Source: CAD feature listing. Evaluate the final solid. Frame: model axes, mm. A direction names the side the tool comes from. Coordinates: 2 decimals unless noted, no trailing zeros. Loops run counter-clockwise (first coordinate to the right, second up) from the corner with the lowest first, then second, coordinate; pieces in that order, holes last.
Item 1: Pin query (flat end, axial travel): pin 1 Ø3 at (y, z) = (-5.5, -1.5) entering from -X; pin 2 Ø12 at (x, y) = (18.5, -10) entering from +Z; pin 3 Ø0.8 at (x, z) = (3.5, 3.5) entering from -Y; pin 4 Ø1.5 at (x, z) = (5.5, -1) entering from +Y. Return the tip coordinate at first contact, or that it passes through.
Item 2: Section query A-A, the plane y = 12.25. Return the cut outline in (x, z).
Item 3: Pull-direction query (X, two-part tool) for faces 1 (the flat face through (30, -3, 6.8)), 2 (the flat face through (0, 0, 0)), 3 (the flat face through (11.091, -8.787, -5.666)); classes: +X half, -X half, draft (parallel to the pull), parting line (faces both ways), or undercut.
Item 4: Section query B-B, the plane z = 4. Return the cut outline in (x, y).
Item 5: Reachability of faces 4 (the flat face through (15, -3, -6.8)), 5 (the flat face through (14, -5, -4.5)), 6 (the flat face through (2, -1, -5.3)), 7 (the flat face through (13, -1, 5.3)), 8 (the flat face through (4, 5.3, 2)) from +Z, -Z, +X, -X, +Y, -Y: full face, straight path, thin tool, end or side. Return the list, or none.
Item 6: Line query: probe 1 along X at (y, z) = (9, -3.25); probe 2 along X at (y, z) = (6.25, 1); probe 3 along X at (y, z) = (-1, 3.25). Output: solid intervals per line, ascending.
Item 7: Section query C-C, the plane y = -11.5. Return the cut outline in (x, z), then the cut area to 3 significant figures.
```python
from build123d import *

# Parameters (mm, degrees)
PAD_DEPTH            = 31
SKETCH001_W          = 11
SKETCH001_H          = 28.2
POCKET_DEPTH         = 10.6
SKETCH002_R          = 3
PAD001_DEPTH         = 3.8
SKETCH003_R          = 1.7
PAD002_DEPTH         = 4.8
SKETCH004_R          = 1.55
POCKET001_DEPTH      = 3.001
POCKET001_DEPTH_BACK = -10.601
POCKET002_DEPTH      = 2.3
SKETCH006_W          = 16
SKETCH006_H          = 28.2
POCKET003_DEPTH      = 1.5
SKETCH007_W          = 24
SKETCH007_H          = 1.2
POCKET004_DEPTH      = 10.6
SKETCH008_W          = 15
SKETCH008_H          = 24.4
POCKET005_DEPTH      = 13.601
SKETCH009_R          = 3
PAD003_DEPTH         = 2
POCKET006_DEPTH      = 3
SKETCH011_R          = 3
PAD004_DEPTH         = 2
POCKET007_DEPTH      = 3


with BuildPart() as part:
    # Sketch → Pad (new body)
    with BuildSketch(Plane.YZ):
        with BuildLine():
            Line((-13.3, 6.8), (-13.3, -6.8))
            Line((-13.3, -6.8), (6.800033, -6.8))
            ThreePointArc((6.800033, -6.8), (13.6, 3.4e-05), (6.799965, 6.8))
            Line((-13.3, 6.8), (6.799965, 6.8))
        make_face()
    extrude(amount=PAD_DEPTH)

    # Sketch001 (on Face4 of Pad) → Pocket (cut)
    with BuildSketch(Plane(origin=(0, 0, 6.8), x_dir=(0, -1, 0), z_dir=(0, 0, 1))):
        with Locations((7.8, 15.5)):
            Rectangle(SKETCH001_W, SKETCH001_H)
    extrude(amount=-POCKET_DEPTH, mode=Mode.SUBTRACT)

    # Sketch002 (on Face7 of Pocket) → Pad001 (join)
    with BuildSketch(Plane(origin=(0, 0, -3.8), x_dir=(0, -1, 0), z_dir=(0, 0, 1))):
        with Locations((6.3, 18.5)):
            Circle(SKETCH002_R)
        with Locations((6.3, 12.5)):
            Circle(SKETCH002_R)
    extrude(amount=PAD001_DEPTH)

    # Sketch003 (on Face7 of Pad001) → Pad002 (join)
    with BuildSketch(Plane(origin=(0, 0, -3.8), x_dir=(0, -1, 0), z_dir=(0, 0, 1))):
        with Locations((6.3, 18.5)):
            Circle(SKETCH003_R)
        with Locations((6.3, 12.5)):
            Circle(SKETCH003_R)
    extrude(amount=PAD002_DEPTH)

    # Sketch004 (on Face7 of Pad002) → Pocket001 (cut, two sides)
    with BuildSketch(Plane(origin=(0, 0, -3.8), x_dir=(0, -1, 0), z_dir=(0, 0, 1))) as pocket001_sk:
        with Locations((6.3, 18.5)):
            Circle(SKETCH004_R)
        with Locations((6.3, 12.5)):
            Circle(SKETCH004_R)
    extrude(amount=-POCKET001_DEPTH, mode=Mode.SUBTRACT)
    extrude(pocket001_sk.sketch, amount=-POCKET001_DEPTH_BACK, mode=Mode.SUBTRACT)

    # Sketch005 (on Face3 of Pocket001) → Pocket002 (cut)
    with BuildSketch(Plane.YX.offset(6.8)):
        Polygon((-3, 18.5), (-4.65, 21.357884), (-7.95, 21.357884), (-9.6, 18.5), (-7.95, 15.642116), (-4.65, 15.642116), align=None)
        Polygon((-3, 12.5), (-4.65, 15.357884), (-7.95, 15.357884), (-9.6, 12.5), (-7.95, 9.642116), (-4.65, 9.642116), align=None)
    extrude(amount=-POCKET002_DEPTH, mode=Mode.SUBTRACT)

    # Sketch006 (on Face5 of Pocket002) → Pocket003 (cut)
    with BuildSketch(Plane(origin=(0, 0, 6.8), x_dir=(0, -1, 0), z_dir=(0, 0, 1))):
        with Locations((-5.7, 15.5)):
            Rectangle(SKETCH006_W, SKETCH006_H)
    extrude(amount=-POCKET003_DEPTH, mode=Mode.SUBTRACT)

    # Sketch007 (on Face30 of Pocket003) → Pocket004 (cut)
    with BuildSketch(Plane(origin=(0, 0, 5.3), x_dir=(0, -1, 0), z_dir=(0, 0, 1))):
        with Locations((1.3, 2)):
            Rectangle(SKETCH007_W, SKETCH007_H)
        with Locations((1.3, 29)):
            Rectangle(SKETCH007_W, SKETCH007_H)
    extrude(amount=-POCKET004_DEPTH, mode=Mode.SUBTRACT)

    # Sketch008 (on Face3 of Pocket004) → Pocket005 (cut, through all)
    with BuildSketch(Plane.YX.offset(6.8)):
        with Locations((6.7, 15.5)):
            Rectangle(SKETCH008_W, SKETCH008_H)
    extrude(amount=-POCKET005_DEPTH, mode=Mode.SUBTRACT)

    # Sketch009 (on Face19 of Pocket005) → Pad003 (join)
    with BuildSketch(Plane.YZ.offset(3.3)):
        with Locations((6.8, 0)):
            Circle(SKETCH009_R)
    extrude(amount=PAD003_DEPTH)

    # Sketch010 (on Face50 of Pad003) → Pocket006 (cut)
    with BuildSketch(Plane.YZ.offset(5.3)):
        with BuildLine():
            Line((5.3, 5.3), (5.3, 0))
            ThreePointArc((5.3, 0), (6.8, -1.5), (8.3, 0))
            Line((8.3, 0), (8.3, 5.3))
            Line((8.3, 5.3), (5.3, 5.3))
        make_face()
    extrude(amount=-POCKET006_DEPTH, mode=Mode.SUBTRACT)

    # Sketch011 (on Face21 of Pocket006) → Pad004 (join)
    with BuildSketch(Plane(origin=(27.7, 0, 0), x_dir=(0, 1, 0), z_dir=(-1, 0, 0))):
        with Locations((6.8, 0)):
            Circle(SKETCH011_R)
    extrude(amount=PAD004_DEPTH)

    # Sketch012 (on Face57 of Pad004) → Pocket007 (cut)
    with BuildSketch(Plane(origin=(25.7, 0, 0), x_dir=(0, 1, 0), z_dir=(-1, 0, 0))):
        with BuildLine():
            ThreePointArc((8.3, 0), (6.8, 1.5), (5.3, -1e-06))
            Line((5.3, -1e-06), (5.3, -5.3))
            Line((5.3, -5.3), (8.3, -5.3))
            Line((8.3, -5.3), (8.3, 0))
        make_face()
    extrude(amount=-POCKET007_DEPTH, mode=Mode.SUBTRACT)


solid = part.part
```
Verdict:
1. pin 1: stops at x = 0
1. pin 2: stops at z = 1
1. pin 3: stops at y = -2.3
1. pin 4: stops at y = 9.79
2. outline: (0, -4.07) - (3.3, -4.07) - (3.3, 4.07) - (0, 4.07) - close; (27.7, -4.07) - (31, -4.07) - (31, 4.07) - (27.7, 4.07) - close
3. face 1: draft
3. face 2: -X half
3. face 3: undercut
4. outline: (0, -13.3) - (1.4, -13.3) - (1.4, 10.7) - (2.6, 10.7) - (2.6, 8.3) - (3.3, 8.3) - (3.3, 12.3) - (0, 12.3) - close; (2.6, -2.3) - (28.4, -2.3) - (28.4, 5.3) - (27.7, 5.3) - (27.7, -0.8) - (3.3, -0.8) - (3.3, 5.3) - (2.6, 5.3) - close; (27.7, 8.3) - (28.4, 8.3) - (28.4, 10.7) - (29.6, 10.7) - (29.6, -13.3) - (31, -13.3) - (31, 12.3) - (27.7, 12.3) - close
5. face 4: -Z, +X, -X, +Y, -Y
5. face 5: -Z
5. face 6: +Z, -Y
5. face 7: +Z, +Y, -Y
5. face 8: +Z
6. probe 1: x = 0 to 1.4, 2.6 to 3.3, 27.7 to 28.4, 29.6 to 31
6. probe 2: x = 0 to 1.4, 29.6 to 31
6. probe 3: x = 0 to 1.4, 2.6 to 28.4, 29.6 to 31
7. outline: (0, -6.8) - (31, -6.8) - (31, 6.8) - (29.6, 6.8) - (29.6, -5.3) - (28.4, -5.3) - (28.4, -3.8) - (2.6, -3.8) - (2.6, -5.3) - (1.4, -5.3) - (1.4, 6.8) - (0, 6.8) - close
7. area: 119 mm2
